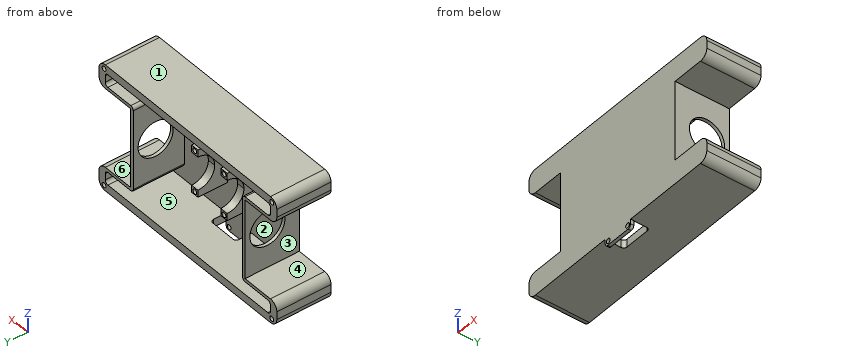
```python
from build123d import *

# Parameters (mm, degrees)
SKETCH1_W           = 177.8
SKETCH1_H           = 101.6
BOSS_EXTRUDE1_DEPTH = 2.54
SKETCH2_W           = 25.4
SKETCH2_H           = 63.5
CUT_EXTRUDE1_DEPTH  = 2.54
SKETCH3_W           = 177.8
SKETCH3_H           = 101.6
SKETCH3_W_2         = 165.1
SKETCH3_H_2         = 88.9
BOSS_EXTRUDE2_DEPTH = 40.64
BOSS_EXTRUDE3_DEPTH = 40.64
SKETCH8_W           = 6.35
SKETCH8_H           = 38.1
BOSS_EXTRUDE4_DEPTH = 10.16
BOSS_EXTRUDE5_DEPTH = 6.35
SKETCH10_W          = 6.35
SKETCH10_H          = 63.5
CUT_EXTRUDE2_DEPTH  = 107.696
SKETCH11_R          = 13.97
CUT_EXTRUDE5_DEPTH  = 2.54
FILLET1_R           = 6.35
FILLET2_R           = 2.54
SKETCH14_W          = 25.4
SKETCH14_H          = 6.35
BOSS_EXTRUDE6_DEPTH = 2.54
SKETCH15_R          = 1.905
CUT_EXTRUDE6_DEPTH  = 8.636
FILLET3_R           = 2.54
SKETCH16_R          = 1.95
CUT_EXTRUDE7_DEPTH  = 10
SKETCH17_R          = 1.905
CUT_EXTRUDE8_DEPTH  = 10
SKETCH18_W          = 25.4
SKETCH18_H          = 12.7
CUT_EXTRUDE9_DEPTH  = 10
FILLET4_R           = 2.54


with BuildPart() as part:
    # Sketch1 → Boss-Extrude1 (new body)
    with BuildSketch(Plane(origin=(0, 0, 0), x_dir=(1, 0, 0), z_dir=(0, 1, 0))):
        Rectangle(SKETCH1_W, SKETCH1_H)
    extrude(amount=BOSS_EXTRUDE1_DEPTH)

    # Sketch2 → Cut-Extrude1 (cut)
    with BuildSketch(Plane(origin=(0, 2.54, 0), x_dir=(1, 0, 0), z_dir=(0, 1, 0))):
        with Locations((-69.85, 0)):
            Rectangle(SKETCH2_W, SKETCH2_H)
        with Locations((69.85, 0)):
            Rectangle(SKETCH2_W, SKETCH2_H)
    extrude(amount=-CUT_EXTRUDE1_DEPTH, mode=Mode.SUBTRACT)

    # Sketch3 → Boss-Extrude2 (add)
    with BuildSketch(Plane(origin=(0, 2.54, 0), x_dir=(1, 0, 0), z_dir=(0, 1, 0))):
        Rectangle(SKETCH3_W, SKETCH3_H)
        Rectangle(SKETCH3_W_2, SKETCH3_H_2, mode=Mode.SUBTRACT)
    extrude(amount=BOSS_EXTRUDE2_DEPTH)

    # Sketch7 → Boss-Extrude3 (add)
    with BuildSketch(Plane(origin=(0, 2.54, 0), x_dir=(1, 0, 0), z_dir=(0, 1, 0))):
        Polygon((-54.61, 34.29), (-82.55, 34.29), (-82.55, 31.75), (-57.15, 31.75), (-57.15, -31.75), (-82.55, -31.75), (-82.55, -34.29), (-54.61, -34.29), align=None)
        Polygon((82.55, 34.29), (54.61, 34.29), (54.61, -34.29), (82.55, -34.29), (82.55, -31.75), (57.15, -31.75), (57.15, 31.75), (82.55, 31.75), align=None)
    extrude(amount=BOSS_EXTRUDE3_DEPTH)

    # Sketch8 → Boss-Extrude4 (add)
    with BuildSketch(Plane(origin=(0, 2.54, 0), x_dir=(1, 0, 0), z_dir=(0, 1, 0))):
        with Locations((-14.605, 0)):
            Rectangle(SKETCH8_W, SKETCH8_H)
    boss_extrude4 = extrude(amount=BOSS_EXTRUDE4_DEPTH)

    # Sketch9 → Boss-Extrude5 (add)
    with BuildSketch(Plane(origin=(-11.43, 0, 0), x_dir=(0, 0, -1), z_dir=(1, 0, 0))):
        with BuildLine():
            Line((-19.05, 26.035), (-19.05, 12.7))
            Line((-19.05, 12.7), (7e-09, 12.7))
            ThreePointArc((7e-09, 12.7), (-9.429268925, 16.60573107), (-13.335, 26.035))
            Line((-13.335, 26.035), (-19.05, 26.035))
        make_face()
        with BuildLine():
            ThreePointArc((13.335, 26.035), (9.42926893, 16.605731075), (7e-09, 12.7))
            Line((7e-09, 12.7), (19.05, 12.7))
            Line((19.05, 12.7), (19.05, 26.035))
            Line((19.05, 26.035), (13.335, 26.035))
        make_face()
    boss_extrude5 = extrude(amount=-BOSS_EXTRUDE5_DEPTH)

    # Sketch10 → Cut-Extrude2 (cut)
    with BuildSketch(Plane(origin=(0, 43.18, 0), x_dir=(1, 0, 0), z_dir=(0, 1, 0))):
        with Locations((-85.725, 0)):
            Rectangle(SKETCH10_W, SKETCH10_H)
        with Locations((85.725, 0)):
            Rectangle(SKETCH10_W, SKETCH10_H)
    extrude(amount=-CUT_EXTRUDE2_DEPTH, mode=Mode.SUBTRACT)

    # Mirror1: Boss-Extrude4, Boss-Extrude5 across plane
    add(boss_extrude4.mirror(Plane(origin=(0, 0, 0), x_dir=(0, 0, 1), z_dir=(1, 0, 0))))
    add(boss_extrude5.mirror(Plane(origin=(0, 0, 0), x_dir=(0, 0, 1), z_dir=(1, 0, 0))))

    # Sketch11 → Cut-Extrude5 (cut)
    with BuildSketch(Plane.ZY.offset(-54.61)):
        with Locations((0, 25.4)):
            Circle(SKETCH11_R)
    cut_extrude5 = extrude(amount=-CUT_EXTRUDE5_DEPTH, mode=Mode.SUBTRACT)

    # Mirror2: Cut-Extrude5 across plane
    add(cut_extrude5.mirror(Plane(origin=(0, 0, 0), x_dir=(0, 0, 1), z_dir=(1, 0, 0))), mode=Mode.SUBTRACT)

    # Fillet1
    fillet1_edges = [part.edges().sort_by_distance(p)[0] for p in [
        (-88.9, 21.59, 31.75),
        (-88.9, 21.59, -31.75),
        (88.9, 21.59, -31.75),
        (88.9, 21.59, 31.75),
        (88.9, 21.59, 50.8),
        (-88.9, 21.59, 50.8),
        (-88.9, 21.59, -50.8),
        (88.9, 21.59, -50.8),
    ]]
    fillet(fillet1_edges, radius=FILLET1_R)

    # Fillet2
    fillet2_edges = [part.edges().sort_by_distance(p)[0] for p in [
        (82.55, 22.86, -34.29),
        (-82.55, 22.86, 44.45),
        (82.55, 22.86, 44.45),
        (82.55, 22.86, -44.45),
        (-82.55, 22.86, -44.45),
        (-54.61, 22.86, 34.29),
        (-54.61, 22.86, -34.29),
        (-82.55, 22.86, -34.29),
        (-82.55, 22.86, 34.29),
        (54.61, 22.86, -34.29),
        (54.61, 22.86, 34.29),
        (82.55, 22.86, 34.29),
    ]]
    fillet(fillet2_edges, radius=FILLET2_R)

    # Sketch14 → Boss-Extrude6 (add)
    with BuildSketch(Plane(origin=(0, 2.54, 0), x_dir=(1, 0, 0), z_dir=(0, 1, 0))):
        with Locations((0, 53.975)):
            Rectangle(SKETCH14_W, SKETCH14_H)
    extrude(amount=-BOSS_EXTRUDE6_DEPTH)

    # Sketch15 → Cut-Extrude6 (cut)
    with BuildSketch(Plane(origin=(0, 2.54, 0), x_dir=(1, 0, 0), z_dir=(0, 1, 0))):
        with Locations(Location((-9.7, 53.975, 0), (0, 0, 270))):
            Circle(SKETCH15_R)
        with Locations(Location((9.7, 53.975, 0), (0, 0, 270))):
            Circle(SKETCH15_R)
    extrude(amount=-CUT_EXTRUDE6_DEPTH, mode=Mode.SUBTRACT)

    # Fillet3
    fillet3_edges = [part.edges().sort_by_distance(p)[0] for p in [
        (-12.7, 1.27, -57.15),
        (12.7, 1.27, -57.15),
    ]]
    fillet(fillet3_edges, radius=FILLET3_R)

    # Sketch16 → Cut-Extrude7 (cut)
    with BuildSketch(Plane(origin=(0, 43.18, 0), x_dir=(1, 0, 0), z_dir=(0, 1, 0))):
        with Locations(Location((-83.82, 46.99, 0), (0, 0, 270))):
            Circle(SKETCH16_R)
        with Locations(Location((83.82, 46.99, 0), (0, 0, 270))):
            Circle(SKETCH16_R)
        with Locations(Location((83.82, -46.99, 0), (0, 0, 270))):
            Circle(SKETCH16_R)
        with Locations(Location((-83.82, -46.99, 0), (0, 0, 270))):
            Circle(SKETCH16_R)
    extrude(amount=-CUT_EXTRUDE7_DEPTH, mode=Mode.SUBTRACT)

    # Sketch17 → Cut-Extrude8 (cut)
    with BuildSketch(Plane(origin=(0, 26.035, 0), x_dir=(1, 0, 0), z_dir=(0, 1, 0))):
        with Locations(Location((-14.605, 16.51, 0), (0, 0, 270))):
            Circle(SKETCH17_R)
        with Locations(Location((14.605, 16.51, 0), (0, 0, 270))):
            Circle(SKETCH17_R)
        with Locations(Location((14.605, -16.51, 0), (0, 0, 270))):
            Circle(SKETCH17_R)
        with Locations(Location((-14.605, -16.51, 0), (0, 0, 270))):
            Circle(SKETCH17_R)
    extrude(amount=-CUT_EXTRUDE8_DEPTH, mode=Mode.SUBTRACT)

    # Sketch18 → Cut-Extrude9 (cut)
    with BuildSketch(Plane(origin=(0, 0, -50.8), x_dir=(-1, 0, 0), z_dir=(0, 0, -1))):
        with Locations((0, 8.89)):
            Rectangle(SKETCH18_W, SKETCH18_H)
    extrude(amount=-CUT_EXTRUDE9_DEPTH, mode=Mode.SUBTRACT)

    # Fillet4
    fillet4_edges = [part.edges().sort_by_distance(p)[0] for p in [
        (12.7, 15.24, -47.625),
        (-12.7, 15.24, -47.625),
    ]]
    fillet(fillet4_edges, radius=FILLET4_R)


solid = part.part
```
Here's how the part is built. I have some questions about the finished solid (model axes, mm). Face numbers are marked on the shaded views. A direction names the side the tool comes from. Give positions to 0.01 mm unless a question says otherwise; leave off trailing zeros. Loops run counter-clockwise (first coordinate to the right, second up) from the corner with the lowest first, then second, coordinate; pieces in that order, holes last. Notation, with made-up numbers: M 32,42 L 53,42 A26 cw 53,80 Z; hole C -16,39.5 d4. An arc over 180 degrees is marked long. Return JSON: item names as keys, results as strings.
Item 1: Imagine slicing it at B-B on z = 16.51. List the corners of the cut face in (x, y) for me (3 decimals), then the cut area to 3 significant figures.
A:
{"outline": "M -57.15,0 L 57.15,0 L 57.15,43.18 L 54.61,43.18 L 54.61,2.54 L 17.78,2.54 L 17.78,26.035 L 16.51,26.035 L 16.51,16.035 L 12.7,16.035 L 12.7,26.035 L 11.43,26.035 L 11.43,2.54 L -11.43,2.54 L -11.43,26.035 L -12.7,26.035 L -12.7,16.035 L -16.51,16.035 L -16.51,26.035 L -17.78,26.035 L -17.78,2.54 L -54.61,2.54 L -54.61,43.18 L -57.15,43.18 Z", "area": "719 mm^2"}
Item 2: Thinking about a two-plate mould opening in X: for the marked faces 1, 2 and 3, which applies, released by +X, released by -X, zero draft, split by the parting line, or undercut?
A:
{"face 1": "zero draft", "face 2": "undercut", "face 3": "released by -X"}
Item 3: On a 3-axis mill with a long thin cutter (end or side, diameter ignored), from which of +Z, -Z, +X, -X, +Y, -Y can I reach the whole of each face in a straight line? I mean the marked faces 4, 5 and 6. Say none if no direction works.
A:
{"face 4": "-X, +Y, -Y", "face 5": "+Y", "face 6": "+X, +Y, -Y"}
Item 4: Imagine slicing it at A-A on x = 1. List the corners of the cut face in (y, z) for me.
A:
{"outline": "M 0,-57.15 L 2.54,-57.15 L 2.54,44.45 L 43.18,44.45 L 43.18,50.8 L 0,50.8 Z; M 15.24,-50.8 L 43.18,-50.8 L 43.18,-44.45 L 15.24,-44.45 Z"}
Item 5: Please list where these lines run through material, in increasing order: line 1 (X direction, y = 21.75, z = -16.51); line 2 (Z direction, x = -68, y = 41.5); line 3 (Z direction, x = -12, y = 4.5).
A:
{"line 1": "x = -57.15 to -54.61, -17.78 to -16.51, -12.7 to -11.43, 11.43 to 12.7, 16.51 to 17.78, 54.61 to 57.15", "line 2": "z = -50.8 to -44.45, -34.29 to -31.75, 31.75 to 34.29, 44.45 to 50.8", "line 3": "z = -19.05 to 19.05, 44.45 to 50.8"}
Item 6: Imagine slicing it at C-C on x = -27. List the corners of the cut face in (y, z) for me.
A:
{"outline": "M 0,-50.8 L 43.18,-50.8 L 43.18,-44.45 L 2.54,-44.45 L 2.54,44.45 L 43.18,44.45 L 43.18,50.8 L 0,50.8 Z"}
Item 7: I'm going to push flat-ended pins straight in: pin 1 Ø7 at (y, z) = (11.5, -3.5) entering from -X; pin 2 Ø2 at (x, z) = (84, 46.5) entering from +Y; pin 3 Ø3 at (x, y) = (9, 32) entering from -Z. Where does each tip first touch, or does it pass through?
A:
{"pin 1": "stops at x = -57.15", "pin 2": "stops at y = 33.18", "pin 3": "stops at z = -50.8"}
Item 8: Imagine slicing it at D-D on z = -4. List the corners of the cut face in (x, y) for me, then the cut area to 3 significant figures.
A:
{"outline": "M -57.15,0 L 57.15,0 L 57.15,12.01 L 54.61,12.01 L 54.61,2.54 L 17.78,2.54 L 17.78,13.31 L 11.43,13.31 L 11.43,2.54 L -11.43,2.54 L -11.43,13.31 L -17.78,13.31 L -17.78,2.54 L -54.61,2.54 L -54.61,12.01 L -57.15,12.01 Z; M -57.15,38.79 L -54.61,38.79 L -54.61,43.18 L -57.15,43.18 Z; M 54.61,38.79 L 57.15,38.79 L 57.15,43.18 L 54.61,43.18 Z", "area": "498 mm^2"}
